CAD build for the part. Positions are in the model's coordinates, mm. Face numbers are marked on the shaded views. A direction names the side the tool comes from. Round coordinates to 2 decimals unless told otherwise and drop trailing zeros. Loops run counter-clockwise (first coordinate to the right, second up) from the corner with the lowest first, then second, coordinate; pieces in that order, holes last. Notation, with made-up numbers: (5.25, 11) - (18.25, 11) arc R28 cw to (18.25, 34) - close; hole circle Ø2 at (89.25, -26). An arc over 180 degrees is marked (long way). Use one line per item in the form item = value.
from build123d import *

# Parameters (mm, degrees)
SKETCH1_W           = 32.385
SKETCH1_H           = 20.32
SKETCH1_R           = 1.5
BOSS_EXTRUDE1_DEPTH = 1.5
SKETCH2_R           = 9
BOSS_EXTRUDE2_DEPTH = 5


with BuildPart() as part:
    # Sketch1 → Boss-Extrude1 (new body)
    with BuildSketch(Plane(origin=(0, 0, 0), x_dir=(1, 0, 0), z_dir=(0, 1, 0))):
        Rectangle(SKETCH1_W, SKETCH1_H)
        with Locations(Location((-13.6925, 7.66, 0), (0, 0, 270))):
            Circle(SKETCH1_R, mode=Mode.SUBTRACT)
        with Locations(Location((13.6925, 7.66, 0), (0, 0, 90))):
            Circle(SKETCH1_R, mode=Mode.SUBTRACT)
        with Locations(Location((13.6925, -7.66, 0), (0, 0, 270))):
            Circle(SKETCH1_R, mode=Mode.SUBTRACT)
        with Locations(Location((-13.6925, -7.66, 0), (0, 0, 90))):
            Circle(SKETCH1_R, mode=Mode.SUBTRACT)
    extrude(amount=BOSS_EXTRUDE1_DEPTH)

    # Sketch2 → Boss-Extrude2 (add)
    with BuildSketch(Plane(origin=(0, 1.5, 0), x_dir=(1, 0, 0), z_dir=(0, 1, 0))):
        with Locations(Location((6.1925, 0, 0), (0, 0, 270))):
            Circle(SKETCH2_R)
    extrude(amount=BOSS_EXTRUDE2_DEPTH)

    # Sketch3 → Revolve1 (revolve)
    with BuildSketch(Plane.XY, mode=Mode.PRIVATE) as revolve1_sk:
        with BuildLine():
            Line((6.1925, 6.5), (6.1925, 16.5))
            Line((6.1925, 16.5), (9.039531448, 16.5))
            ThreePointArc((9.039531448, 16.5), (10.670922292, 15.894350526), (11.51187233, 14.370851132))
            Line((11.51187233, 14.370851132), (12.6925, 6.5))
            Line((12.6925, 6.5), (6.1925, 6.5))
        make_face()
    revolve(revolve1_sk.sketch.rotate(Axis((6.1925, 6.5, 0), (0, 1, 0)), 90), axis=Axis((6.1925, 6.5, 0), (0, 1, 0)))


solid = part.part
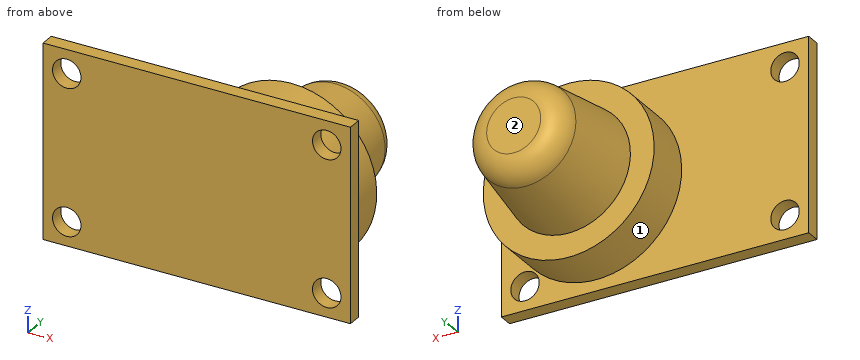
1) Flat gauge pins, fed straight in: pin 1 (6 mm diameter, centred on y = 8, z = 6.5, fed in from +X); pin 2 (1 mm diameter, centred on x = -10.5, z = -4, fed in from +Y); pin 3 (3.5 mm diameter, centred on x = 13.69, z = -7.66, fed in from +Y). Where does each tip first touch, or does it go through?
Report:
pin_1 = 14.3
pin_2 = 1.5
pin_3 = 6.5
2) Slice it at C-C (y = 4). Write the cut outline in (x, z), plus the area to 3 significant figures.
Report:
outline = circle Ø18 at (6.19, 0)
area = 254 mm^2
3) Slice it at B-B (z = 0). Write the cut outline in (x, y).
Report:
outline = (-16.19, 0) - (16.19, 0) - (16.19, 1.5) - (15.19, 1.5) - (15.19, 6.5) - (12.69, 6.5) - (11.51, 14.37) arc R2.5 ccw to (9.04, 16.5) - (3.35, 16.5) arc R2.5 ccw to (0.87, 14.37) - (-0.31, 6.5) - (-2.81, 6.5) - (-2.81, 1.5) - (-16.19, 1.5) - close
4) Tool access for the marked faces 1 and 2: list every direction of +Z, -Z, +X, -X, +Y, -Y with a clear straight run to the whole face (end or side of a thin tool).
Report:
face_1 = +Y
face_2 = +Z, -Z, +X, -X, +Y
5) Slice it at A-A (z = -7.66). Write the cut outline in (x, y).
Report:
outline = (-16.19, 0) - (-15.19, 0) - (-15.19, 1.5) - (-16.19, 1.5) - close; (-12.19, 0) - (12.19, 0) - (12.19, 1.5) - (10.92, 1.5) - (10.92, 6.5) - (1.47, 6.5) - (1.47, 1.5) - (-12.19, 1.5) - close; (15.19, 0) - (16.19, 0) - (16.19, 1.5) - (15.19, 1.5) - close
6) Drill centre lines: probe 1 along X at (y, z) = (0.85, -7.66); probe 2 along Y at (x, z) = (15, -5.25); probe 3 along Z at (x, y) = (6.5, 4). Where is each one in solid material? Low to high.
Report:
probe_1 = -16.19 to -15.19, -12.19 to 12.19, 15.19 to 16.19
probe_2 = 0 to 1.5
probe_3 = -8.99 to 8.99
7) Slice it at D-D (x = -4.5). Write the cut outline in (y, z), plus the area to 3 significant figures.
Report:
outline = (0, -10.16) - (1.5, -10.16) - (1.5, 10.16) - (0, 10.16) - close
area = 30.5 mm^2
